Model file for the job. Use its own axes, mm. A direction names the side the tool comes from. Coordinates: 2 decimals unless noted, no trailing zeros. Write each loop counter-clockwise with the first axis right and the second up, starting at its lowest first coordinate (ties: lowest second). Pieces come first, ordered by that corner, then holes. Notation, with made-up numbers: M -29.75,74.25 L 28.25,74.25 A15 ccw 28.25,95.25 Z; hole C 80.25,11.5 d5. An arc over 180 degrees is marked long. Put each result on its own line as item: value. Start each with the question number.
Q1. Cut at C-C (y = -10). Write the cut outline in (x, z).
Q2. Which spindle directions (+Z, -Z, +X, -X, +Y, -Y) get a long thin tool onto all of the face, cutting with end or side? Do faces 4 (the flat face through (-15, -39, 3)), 5 (the cylindrical face through (-0.09, -46.75, 2.59)), 6 (the flat face through (28, -24.5, 3)). Say none if no direction does.
Q3. Drill centre lines: line 1 along Y through (x, z) = (-30, 2.35); line 2 along X through (y, z) = (-3, 2.7); line 3 along Y through (x, z) = (-12, 3.8). Where is each one in solid material? Low to high.
Q4. Pull direction Y, two halves, no side cores. Call faces 1 (the flat face through (25, -10, 3)), 2 (the flat face through (0, 0, 3)), 3 (the cylindrical face through (-28.092, -18.899, 2.835)): pulls with the +Y half, pulls with the -Y half, needs draft (parallel to the pull), parting line crosses it, or undercut.
Q5. Drop flat-ended pins along their axis: pin 1 (3 mm diameter, centred on x = -28, z = 1.5, fed in from +Y); pin 2 (5 mm diameter, centred on x = 0, y = -42, fed in from +Z); pin 3 (1.6 mm diameter, centred on y = -11, z = 1.5, fed in from +X); pin 4 (1 mm diameter, centred on x = 26, z = 2.5, fed in from -Y). Give the stop position or say it passes through.
Q6. Cut at A-A (z = 0.75). Give the number of separate pieces and of enclosed holes in the cut face, then the cut area to 3 significant figures.
Q7. Cut at B-B (x = 0). Write the cut outline in (y, z), then the cut area to 3 significant figures.
```python
from build123d import *

# Parameters (mm, degrees)
SKETCH1_R           = 3
SKETCH1_R_2         = 2
SKETCH1_R_3         = 2.75
BOSS_EXTRUDE1_DEPTH = 5.75
CHAMFER1_SIZE       = 0.5


with BuildPart() as part:
    # Sketch1 → Boss-Extrude1 (new body)
    with BuildSketch(Plane.XY):
        with BuildLine():
            Line((19, 0), (-19, 0))
            ThreePointArc((-19, 0), (-23.242640687, -1.757359313), (-25, -6))
            Line((-25, -6), (-25, -13.5))
            ThreePointArc((-25, -13.5), (-25.292893219, -14.207106781), (-26, -14.5))
            Line((-26, -14.5), (-30, -14.5))
            ThreePointArc((-30, -14.5), (-35, -19.5), (-30, -24.5))
            Line((-30, -24.5), (-26, -24.5))
            ThreePointArc((-26, -24.5), (-25.292893219, -24.792893219), (-25, -25.5))
            Line((-25, -25.5), (-25, -33))
            ThreePointArc((-25, -33), (-23.242640687, -37.242640687), (-19, -39))
            Line((-19, -39), (-10.322911411, -39))
            ThreePointArc((-10.322911411, -39), (-6.72058658, -40.201744503), (-4.561286437, -43.325581395))
            ThreePointArc((-4.561286437, -43.325581395), (0, -46.75), (4.561286437, -43.325581395))
            ThreePointArc((4.561286437, -43.325581395), (6.72058658, -40.201744503), (10.322911411, -39))
            Line((10.322911411, -39), (19, -39))
            ThreePointArc((19, -39), (23.242640687, -37.242640687), (25, -33))
            Line((25, -33), (25, -25.5))
            ThreePointArc((25, -25.5), (25.292893219, -24.792893219), (26, -24.5))
            Line((26, -24.5), (30, -24.5))
            ThreePointArc((30, -24.5), (35, -19.5), (30, -14.5))
            Line((30, -14.5), (26, -14.5))
            ThreePointArc((26, -14.5), (25.292893219, -14.207106781), (25, -13.5))
            Line((25, -13.5), (25, -6))
            ThreePointArc((25, -6), (23.242640687, -1.757359313), (19, 0))
        make_face()
        with Locations((20, -5)):
            Circle(SKETCH1_R, mode=Mode.SUBTRACT)
        with Locations((30, -19.5)):
            Circle(SKETCH1_R_2, mode=Mode.SUBTRACT)
        with Locations((-30, -19.5)):
            Circle(SKETCH1_R_2, mode=Mode.SUBTRACT)
        with Locations((0, -42)):
            Circle(SKETCH1_R_3, mode=Mode.SUBTRACT)
        with Locations((-20, -5)):
            Circle(SKETCH1_R, mode=Mode.SUBTRACT)
    extrude(amount=BOSS_EXTRUDE1_DEPTH)

    # Chamfer1
    chamfer1_edges = [part.edges().sort_by_distance(p)[0] for p in [
        (35, -19.5, 5.75),
        (28, -14.5, 5.75),
        (25.292893219, -14.207106781, 5.75),
        (25, -9.75, 5.75),
        (23.242640687, -1.757359313, 5.75),
        (0, 0, 5.75),
        (-23.242640687, -1.757359313, 5.75),
        (-25, -9.75, 5.75),
        (-25.292893219, -14.207106781, 5.75),
        (-28, -14.5, 5.75),
        (-35, -19.5, 5.75),
        (-28, -24.5, 5.75),
        (-25.292893219, -24.792893219, 5.75),
        (-25, -29.25, 5.75),
        (-23.242640687, -37.242640687, 5.75),
        (-14.661455706, -39, 5.75),
        (-6.72058658, -40.201744503, 5.75),
        (0, -46.75, 5.75),
        (6.72058658, -40.201744503, 5.75),
        (14.661455706, -39, 5.75),
        (23.242640687, -37.242640687, 5.75),
        (25, -29.25, 5.75),
        (25.292893219, -24.792893219, 5.75),
        (28, -24.5, 5.75),
    ]]
    chamfer(chamfer1_edges, length=CHAMFER1_SIZE)


solid = part.part
```
Computed values:
1. outline: M -25,0 L 25,0 L 25,5.25 L 24.5,5.75 L -24.5,5.75 L -25,5.25 Z
2. face 4: +Z, -Z, -X, -Y
2. face 5: +Z, -Z, -Y
2. face 6: +Z, -Z, +X, -Y
3. line 1: -24.5 to -21.5, -17.5 to -14.5
3. line 2: -24.2 to -22.24, -17.76 to 17.76, 22.24 to 24.2
3. line 3: -39 to 0
4. face 1: needs draft
4. face 2: pulls with the +Y half
4. face 3: undercut
5. pin 1: y = -14.5
5. pin 2: through
5. pin 3: x = 25
5. pin 4: y = -24.63
6. separate pieces: 1
6. enclosed holes: 5
6. area: 2,070 mm2
7. outline: M -46.75,0 L -44.75,0 L -44.75,5.75 L -46.25,5.75 L -46.75,5.25 Z; M -39.25,0 L 0,0 L 0,5.25 L -0.5,5.75 L -39.25,5.75 Z
7. area: 237 mm2
